Verification items for this drawing (mm, ordinates from the low corner). A direction names the side the tool comes from. Round coordinates to 2 decimals unless told otherwise and drop trailing zeros. Loops run counter-clockwise (first coordinate to the right, second up) from the corner with the lowest first, then second, coordinate; pieces in that order, holes last. Notation, with made-up numbers: M 72,40 L 97,40 A11 ccw 97,61 Z; hole C 22.5,-24 d11. An arc over 180 degrees is marked long. Answer in a Markdown table with one row per item. Add a question column.
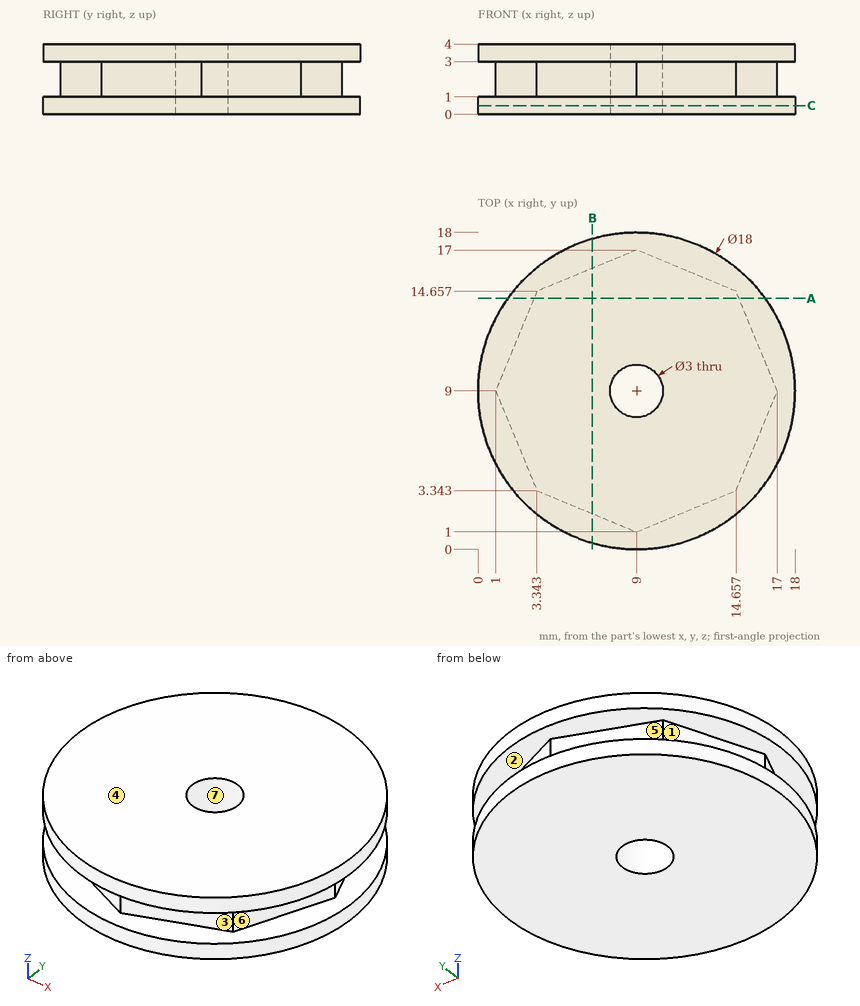
1) Go/stop test with a flat-tipped pin: pin 1 (3.5 mm diameter, centred on x = 9, y = 9, fed in from -Z). Record where the tip stops, or that it passes through.
2) Set-up check for the marked faces 1, 2, 3 and 4: record each of +Z, -Z, +X, -X, +Y, -Y from which the full face is reachable in a straight line by a thin tool's end or side.
3) Draft check along Y on the marked faces 5, 6 and 7. Enter one of: +Y half, -Y half, draft (parallel to the pull), parting line (faces both ways), or undercut.
4) Cross-section at B-B, the plane x = 6.5. Record the boundary of the cut face in (y, z).
5) Cross-section at C-C, the plane z = 0.5. Record the boundary of the cut face in (x, y).
6) Thickness scan on L1, parallel to Z at x = 1, y = 6.75; L2, parallel to Y at x = 14, z = 2.5; L3, parallel to Y at x = 5.5, z = 1.35. Record the ranges inside material, lowest first. Write a range as [from, to].
7) Cross-section at A-A, the plane y = 14.25. Record the boundary of the cut face in (x, z).
Worked answers:
| question | item | result |
|---|---|---|
| 1 | pin 1 | stops at z = 0 |
| 2 | face 1 | -X, +Y |
| 2 | face 2 | none |
| 2 | face 3 | +X, -Y |
| 2 | face 4 | +Z, +X, -X, +Y, -Y |
| 3 | face 5 | +Y half |
| 3 | face 6 | -Y half |
| 3 | face 7 | undercut |
| 4 | outline | M 0.35,0 L 17.65,0 L 17.65,1 L 15.96,1 L 15.96,3 L 17.65,3 L 17.65,4 L 0.35,4 L 0.35,3 L 2.04,3 L 2.04,1 L 0.35,1 Z |
| 5 | outline | C 9,9 d18; hole C 9,9 d3 |
| 6 | L1 | z = [0, 1], [3, 4] |
| 6 | L2 | y = [3.07, 14.93] |
| 6 | L3 | y = [2.45, 15.55] |
| 7 | outline | M 1.69,0 L 16.31,0 L 16.31,1 L 14.83,1 L 14.83,3 L 16.31,3 L 16.31,4 L 1.69,4 L 1.69,3 L 3.17,3 L 3.17,1 L 1.69,1 Z |
